Geometry: final body of the model. Coordinates: model frame, mm. A direction names the side the tool comes from. Give positions to 0.01 mm unless a question says otherwise; leave off trailing zeros. Order: outer loops, then holes, each group sorted by start corner. A loop starts at its lowest first (then second) coordinate and runs counter-clockwise, first axis right, second up. Notation, with made-up numbers: (-2.5, -4) - (31.5, -4) arc R13 ccw to (31.5, 12) - close; hole circle Ø10 at (46, 83.25). An arc over 180 degrees is marked (long way). Put each result on its own line as item: value. Start each with the question number.
1. Section B-B on y = -55. Return the cut outline in (x, z).
2. Section C-C on z = 10.75. Return the cut outline in (x, y).
3. First-contact query: P1, Ø8, axis at x = -17, z = 24.6, coming from the +Y side; P2, Ø3.5, axis at y = -55, z = 23, coming from the +X side; P3, Ø8, axis at x = -17, z = 24.6, coming from the -Y side. Flat tips, straight axial feed; report the tip coordinate or a pass-through.
4. Ray query, line 1 along Z through (x, y) = (-26.1, -20); line 2 along Z through (x, y) = (-17, -7.7); line 3 along Y through (x, z) = (-6.75, 10). Return the intervals inside material, ascending. Write a range as from..to.
5. Mould query, pull axis Y, two halves, no side actions, for faces 4 (the cylindrical face through (-27.54, -56.48, 6.39)), 5 (the cylindrical face through (-14.452, 2.535, 5.512)), 6 (the flat face through (-15, 5, 15)). Classes: pulls with the +Y half, pulls with the -Y half, needs draft (parallel to the pull), parting line crosses it, or undercut.
6. Section D-D on x = -27.25. Return the cut outline in (y, z), plus the area to 3 significant figures.
7. Set-up query: faces 1 (the flat face through (-25.2, -12.6, 30)), 2 (the flat face through (-13, -10.2, 15)), 3 (the flat face through (-13, 0, 15)). Return all of +Z, -Z, +X, -X, +Y, -Y with unobstructed straight access to the full face (end or side cutting, diameter ignored); none if empty.
8. Section A-A on x = -17. Return the cut outline in (y, z), plus the area to 3 significant figures.
from build123d import *

# Parameters (mm, degrees)
BOSS_EXTRUDE1_DEPTH = 30
CUT_EXTRUDE1_REACH  = 75.485
SKETCH2_R           = 1.6
SKETCH3_R           = 2.55
CUT_EXTRUDE2_DEPTH  = 78.620873481


with BuildPart() as part:
    # Sketch1 → Boss-Extrude1 (new body)
    with BuildSketch(Plane.XY):
        Polygon((0, 0), (0, 5), (-30, 5), (-30, -60), (-25, -60), (-25, -10.2), (0, -10.2), (0, -5.2), (-25, -5.2), (-25, 0), align=None)
    extrude(amount=BOSS_EXTRUDE1_DEPTH)

    # Sketch2 → Cut-Extrude1 (cut, up to next)
    with BuildSketch(Plane.ZY.offset(30), mode=Mode.PRIVATE) as cut_extrude1_sk1:
        with Locations(Location((7, -20, 0), (0, 0, 270))):
            Circle(SKETCH2_R)
    cut_extrude1_tool1 = extrude(cut_extrude1_sk1.sketch, amount=-CUT_EXTRUDE1_REACH, mode=Mode.PRIVATE) & part.part
    # Sketch2 → Cut-Extrude1 (cut, up to next)
    with BuildSketch(Plane.ZY.offset(30), mode=Mode.PRIVATE) as cut_extrude1_sk2:
        with Locations(Location((23, -20, 0), (0, 0, 270))):
            Circle(SKETCH2_R)
    cut_extrude1_tool2 = extrude(cut_extrude1_sk2.sketch, amount=-CUT_EXTRUDE1_REACH, mode=Mode.PRIVATE) & part.part
    # Sketch2 → Cut-Extrude1 (cut, up to next)
    with BuildSketch(Plane.ZY.offset(30), mode=Mode.PRIVATE) as cut_extrude1_sk3:
        with Locations(Location((7, -55, 0), (0, 0, 270))):
            Circle(SKETCH2_R)
    cut_extrude1_tool3 = extrude(cut_extrude1_sk3.sketch, amount=-CUT_EXTRUDE1_REACH, mode=Mode.PRIVATE) & part.part
    # Sketch2 → Cut-Extrude1 (cut, up to next)
    with BuildSketch(Plane.ZY.offset(30), mode=Mode.PRIVATE) as cut_extrude1_sk4:
        with Locations(Location((23, -55, 0), (0, 0, 270))):
            Circle(SKETCH2_R)
    cut_extrude1_tool4 = extrude(cut_extrude1_sk4.sketch, amount=-CUT_EXTRUDE1_REACH, mode=Mode.PRIVATE) & part.part
    add(cut_extrude1_tool1.solids().sort_by_distance((-30, -20, 7))[0], mode=Mode.SUBTRACT)
    add(cut_extrude1_tool2.solids().sort_by_distance((-30, -20, 23))[0], mode=Mode.SUBTRACT)
    add(cut_extrude1_tool3.solids().sort_by_distance((-30, -55, 7))[0], mode=Mode.SUBTRACT)
    add(cut_extrude1_tool4.solids().sort_by_distance((-30, -55, 23))[0], mode=Mode.SUBTRACT)

    # Sketch3 → Cut-Extrude2 (cut, through all)
    with BuildSketch(Plane(origin=(0, 5, 0), x_dir=(1, 0, 0), z_dir=(0, 1, 0))):
        with Locations(Location((-17, -5.4, 0), (0, 0, 180))):
            Circle(SKETCH3_R)
        with Locations(Location((-17, -24.6, 0), (0, 0, 180))):
            Circle(SKETCH3_R)
    extrude(amount=-CUT_EXTRUDE2_DEPTH, mode=Mode.SUBTRACT)


solid = part.part
Resolved:
1. outline: (-30, 0) - (-25, 0) - (-25, 5.4) - (-30, 5.4) - close; (-30, 8.6) - (-25, 8.6) - (-25, 21.4) - (-30, 21.4) - close; (-30, 24.6) - (-25, 24.6) - (-25, 30) - (-30, 30) - close
2. outline: (-30, -60) - (-25, -60) - (-25, -10.2) - (0, -10.2) - (0, -5.2) - (-25, -5.2) - (-25, 0) - (0, 0) - (0, 5) - (-30, 5) - close
3. P1: y = 5
3. P2: x = -25
3. P3: y = -10.2
4. line 1: 0..5.4, 8.6..21.4, 24.6..30
4. line 2: 0..2.85, 7.95..22.05, 27.15..30
4. line 3: -10.2..-5.2, 0..5
5. face 4: undercut
5. face 5: needs draft
5. face 6: pulls with the +Y half
6. outline: (-60, 0) - (5, 0) - (5, 30) - (-60, 30) - close; hole circle Ø3.2 at (-55, 7); hole circle Ø3.2 at (-55, 23); hole circle Ø3.2 at (-20, 7); hole circle Ø3.2 at (-20, 23)
6. area: 1,920 mm^2
7. face 1: +Z, +X, -X, +Y, -Y
7. face 2: +Z, -Z, +X, -Y
7. face 3: +Z, -Z, +X
8. outline: (-10.2, 0) - (-5.2, 0) - (-5.2, 2.85) - (-10.2, 2.85) - close; (-10.2, 7.95) - (-5.2, 7.95) - (-5.2, 22.05) - (-10.2, 22.05) - close; (-10.2, 27.15) - (-5.2, 27.15) - (-5.2, 30) - (-10.2, 30) - close; (0, 0) - (5, 0) - (5, 2.85) - (0, 2.85) - close; (0, 7.95) - (5, 7.95) - (5, 22.05) - (0, 22.05) - close; (0, 27.15) - (5, 27.15) - (5, 30) - (0, 30) - close
8. area: 198 mm^2
